Source: CAD feature listing. Evaluate the final solid. Frame: model axes, mm. Give positions to 0.01 mm unless a question says otherwise; leave off trailing zeros. Write each loop counter-clockwise with the first axis right and the second up, starting at its lowest first coordinate (ties: lowest second). Pieces come first, ordered by that corner, then holes. Notation, with made-up numbers: (9, 71.5) -> (24, 71.5) arc R25 cw to (24, 85.5) -> close; hole circle Ø6 at (-38, 3.25). An arc over 180 degrees is marked (long way). Write item = value, one per line.
Autodesk Inventor part; units mm, degrees
ref_plane "YZ Plane" through (0, 0, 0) normal (1, 0, 0) x (0, 1, 0)
ref_plane "XZ Plane" through (0, 0, 0) normal (0, 1, 0) x (-1, 0, 0)
ref_plane "XY Plane" through (0, 0, 0) normal (0, 0, 1) x (1, 0, 0)
sketch "Sketch1" plane through (0, 0, 0) normal (0, 0, 1) x (1, 0, 0)
  circle A0 centre (0, 0) radius 5.7
  dimension "d0" = 11.4
extrude "Extrusion1" add sketch "Sketch1" along normal blind 16
chamfer "Chamfer1" distance 0.8 angle 45 1 edges at (-5.7, 0, 16)
sketch "Sketch2" plane through (0, 0, 0) normal (0, 0, 1) x (1, 0, 0)
  circle A0 centre (0, 0) radius 2.9
  dimension "d6" = 5.8
extrude "Extrusion2" cut sketch "Sketch2" along normal up to surface (16 mm away)
properties part number "Insert16mm"
(1) Section query A-A (y = 0). Return loops of the section in (x, z).
Values follow:
outline = (-5.7, 0) -> (-2.9, 0) -> (-2.9, 16) -> (-4.9, 16) -> (-5.7, 15.2) -> close; (2.9, 0) -> (5.7, 0) -> (5.7, 15.2) -> (4.9, 16) -> (2.9, 16) -> close
(2) First-contact query: pin 1 (6 mm diameter, centred on y = -3.5, z = 8, fed in from -X); pin 2 (3.5 mm diameter, centred on x = 0, y = 0, fed in from +Z); pin 3 (6 mm diameter, centred on y = 4.5, z = 7.5, fed in from +X); pin 4 (2 mm diameter, centred on y = -4, z = 12.5, fed in from +X). Flat tips, straight axial feed; report the tip coordinate or a pass-through.
Values follow:
pin_1 = -5.68
pin_2 = through
pin_3 = 5.5
pin_4 = 4.85
(3) Pull-direction query (X, two-part tool) for faces 1 (the face through (-2.9, -0.1, 7.9)), 2 (the face through (-0.1, -3.2, 16)), 3 (the face through (-4.5, 3.5, 7.5)); classes: pulls with the +X half, pulls with the -X half, needs draft (parallel to the pull), parting line crosses it, or undercut.
Values follow:
face_1 = undercut
face_2 = needs draft
face_3 = parting line crosses it
(4) Section query C-C (z = 3.25). Return loops of the section in (x, y), plus the area to 3 significant figures.
Values follow:
outline = circle Ø11.4 at (0, 0); hole circle Ø5.8 at (0, 0)
area = 75.6 mm2
(5) Material intervals for line 1 (Y direction, x = 0, z = 7.5); line 2 (X direction, y = -1.25, z = 4.5); line 3 (X direction, y = -0.25, z = 6.75), sorted ascending.
Values follow:
line_1 = -5.7 to -2.9, 2.9 to 5.7
line_2 = -5.56 to -2.62, 2.62 to 5.56
line_3 = -5.69 to -2.89, 2.89 to 5.69
